```python
from build123d import *


# Not quite as in the source:
# - ends of sketch curves that miss each other by under 0.0002 mm in the source are joined


with BuildPart() as f1:
    # F0 (on Front) → F1 (revolve)
    with BuildSketch(Plane.XZ):
        Polygon((-7, 0), (0, 0), (0, 1.3), (-7.3899972171, 1.3), align=None)
        Polygon((-9, 0), (-7, 0), (-7.3899972171, 1.3), (-9, 1.3), align=None)
        Polygon((-10.4999892964, 4.9999928643), (-9, 0), (-9, 1.3), (-7.3899972171, 1.3), (-8.4999892965, 5), (-9.4999892964, 4.9999964322), align=None)
        Polygon((-9.4999892964, 4.9999964322), (-8.4999892965, 5), (-8.4999964322, 7), (-9.4999964321, 6.9999964322), align=None)
        Polygon((-9.4999964321, 6.9999964322), (-8.4999964322, 7), (-8.5, 8), (-9.4999964321, 8), align=None)
        Polygon((-14.5, 7), (-9.4999964321, 7), (-9.4999964321, 7.9999964322), (-14.5, 8), align=None)
    revolve(axis=Axis((0, 0, 0.65), (0, 0, 1)))


solid = f1.part
```
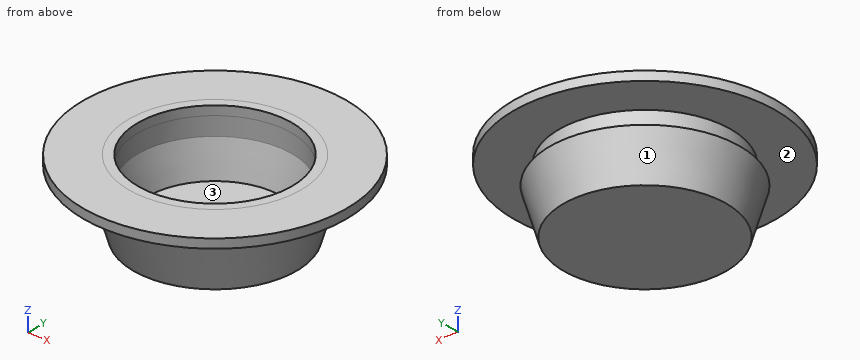
Model file for the job. Use its own axes, mm. Face numbers are marked on the shaded views. Coordinates: 2 decimals unless noted, no trailing zeros. Loops run counter-clockwise (first coordinate to the right, second up) from the corner with the lowest first, then second, coordinate; pieces in that order, holes last. Notation, with made-up numbers: (20.5, 48.25) - (74.5, 48.25) arc R30 ccw to (74.5, 86.25) - close; hole circle Ø11 at (-4, 76.5). An arc over 180 degrees is marked (long way). Write item = value, one per line. Start each with the question number.
Item 1: Saw through at C-C, the plane z = 3. List the corners of the cut face in (x, y), then the cut area to 3 significant figures.
Item 2: Saw through at B-B, the plane z = 6.25. List the corners of the cut face in (x, y).
Item 3: Wall check: probe 1 along Y at (x, z) = (0, 7.7); probe 2 along Y at (x, z) = (0, 6.1). Give the ranges that are in metal, low to high. Write a range as [from, to].
Item 4: Pull direction X, two halves, no side cores. Call the marked faces 1, 2 and 3: +X half, -X half, draft (parallel to the pull), parting line (faces both ways), or undercut.
Item 5: Drop a flat-ended pin along its axis: pin 1 Ø3 at (y, z) = (3.5, 2) entering from +X. Give the stop position or say it passes through.
Answers:
q1.outline = circle Ø19.8 at (0, 0); hole circle Ø15.8 at (0, 0)
q1.area = 112 mm2
q2.outline = circle Ø19 at (0, 0); hole circle Ø17 at (0, 0)
q3.probe_1 = [-14.5, -8.5], [8.5, 14.5]
q3.probe_2 = [-9.5, -8.5], [8.5, 9.5]
q4.face_1 = parting line
q4.face_2 = draft
q4.face_3 = undercut
q5.pin_1 = 9.62
